CAD build for the part. Positions are in the model's coordinates, mm. Round coordinates to 2 decimals unless told otherwise and drop trailing zeros. Loops run counter-clockwise (first coordinate to the right, second up) from the corner with the lowest first, then second, coordinate; pieces in that order, holes last. Notation, with made-up numbers: M -26.5,50 L 8.5,50 A30 ccw 8.5,76 Z; hole C 39,40.25 d7. An arc over 180 degrees is marked long. One line per item, written item: value. Start each with the question number.
from build123d import *

# Parameters (mm, degrees)
EXTRUDE_1_DEPTH = 2
HOLE_WIZARD_1_D = 1.3
FILLET_1_R      = 2


with BuildPart() as part:
    # 草图1 → 凸台-拉伸1 (new, symmetric)
    with BuildSketch(Plane.XY):
        Polygon((-3.464101615, 0), (-9.8, 0), (-9.8, -4.8), (9.8, -4.8), (9.8, 0), (3.464101615, 0), align=None)
    extrude(amount=EXTRUDE_1_DEPTH, both=True)

    # 孔1 (through all)
    with Locations(Plane(origin=(0, 0, 0), x_dir=(1, 0, 0), z_dir=(0, 1, 0))):
        with Locations((-5.65, 0), (5.65, 0)):
            Hole(HOLE_WIZARD_1_D / 2)

    # 草图5 → 切除-旋转1 (revolve, cut)
    with BuildSketch(Plane.XY):
        with BuildLine():
            Line((0, -8.95), (0, -4.8))
            Line((0, -4.8), (0, -0.65))
            ThreePointArc((0, -0.65), (-4.15, -4.8), (0, -8.95))
        make_face()
    revolve(axis=Axis((0, 0, 0), (0, -1, 0)), mode=Mode.SUBTRACT)

    # 圆角1
    fillet_1_edges = [part.edges().sort_by_distance(p)[0] for p in [
        (9.8, 0, 0),
        (-9.8, 0, 0),
    ]]
    fillet(fillet_1_edges, radius=FILLET_1_R)


solid = part.part
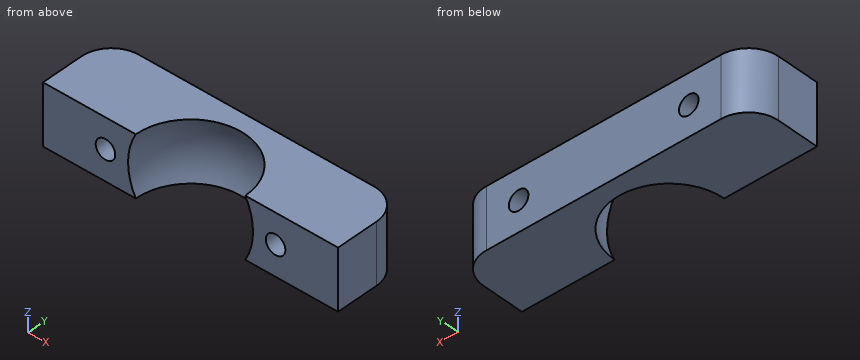
(1) Flat gauge pins, fed straight in: P1, Ø1, axis at y = -1, z = 0, coming from the -X side; P2, Ø2, axis at x = 2.5, z = 0.5, coming from the -Y side. Where does each tip first touch, or does it go through?
(2) Slice it at A-A, the plane x = 5.65. List the corners of the cut face in (y, z), and give its area (3 significant figures).
(3) Slice it at D-D, the plane y = -1.1. List the corners of the cut face in (x, z), and give its area (3 significant figures).
(4) Slice it at B-B, the plane y = -3.45. List the corners of the cut face in (x, z).
(5) Slice it at C-C, the plane z = 0. List the corners of the cut face in (x, y), and give its area (3 significant figures).
(6) Probe L1, parallel to X at y = -1.8, z = 0.2; L2, parallel to Z at x = 5.65, y = -1.35; L3, parallel to X at y = -1.1, z = -0.3. List the from-to ranges inside material, lowest first.
Check result:
1. P1: stops at x = -9.74
1. P2: stops at y = -2.65
2. outline: M -4.8,-2 L 0,-2 L 0,-0.65 L -4.8,-0.65 Z; M -4.8,0.65 L 0,0.65 L 0,2 L -4.8,2 Z
2. area: 13.0 mm^2
3. outline: M -9.59,-2 L 9.59,-2 L 9.59,2 L -9.59,2 Z; hole C -5.65,0 d1.3; hole C 0,0 d3.76; hole C 5.65,0 d1.3
3. area: 62.9 mm^2
4. outline: M -9.8,-2 L -3.38,-2 A3.92 cw -3.38,2 L -9.8,2 Z; M 3.38,-2 L 9.8,-2 L 9.8,2 L 3.38,2 A3.92 cw Z; hole C -5.65,0 d1.3; hole C 5.65,0 d1.3
5. outline: M -9.8,-4.8 L -6.3,-4.8 L -6.3,0 L -7.8,0 A2 ccw -9.8,-2 Z; M -5,-4.8 L -4.15,-4.8 A4.15 cw 4.15,-4.8 L 5,-4.8 L 5,0 L -5,0 Z; M 6.3,-4.8 L 9.8,-4.8 L 9.8,-2 A2 ccw 7.8,0 L 6.3,0 Z
5. area: 52.8 mm^2
6. L1: x = -9.79 to -6.27, -5.03 to -2.86, 2.86 to 5.03, 6.27 to 9.79
6. L2: z = -2 to -0.65, 0.65 to 2
6. L3: x = -9.59 to -6.23, -5.07 to -1.86, 1.86 to 5.07, 6.23 to 9.59
